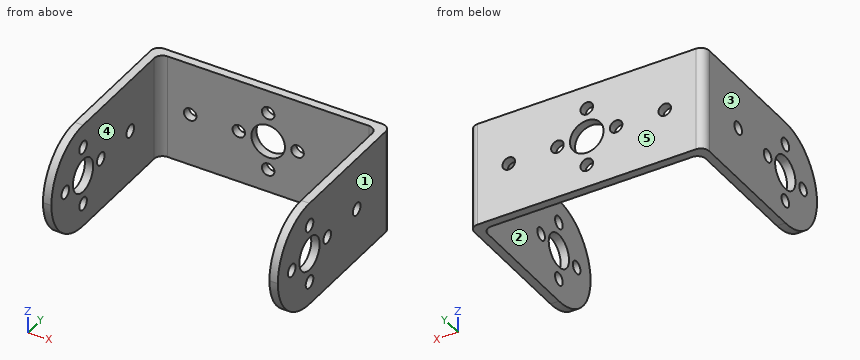
from build123d import *

# Parameters (mm, degrees)
SKETCH_1_W          = 52
SKETCH_1_H          = 25
SKETCH_1_R          = 4
SKETCH_1_R_2        = 1.5
EXTRUDE_1_DEPTH     = 2
SKETCH_2_W          = 2
SKETCH_2_H          = 25
EXTRUDE_2_DEPTH     = 44.5
FILLET_1_R          = 12.5
FILLET_2_R          = 12.5
SKETCH_3_R          = 4
SKETCH_3_R_2        = 1.5
CUT_EXTRUDE_1_DEPTH = 64.5
FILLET_5_R          = 2


with BuildPart() as part:
    # 草图1 → 凸台-拉伸1 (new body)
    with BuildSketch(Plane(origin=(0, 0, 0), x_dir=(1, 0, 0), z_dir=(0, 1, 0))):
        with Locations((-26, 12.5)):
            Rectangle(SKETCH_1_W, SKETCH_1_H)
        with Locations(Location((-26, 12.5, 0), (0, 0, 270))):
            Circle(SKETCH_1_R, mode=Mode.SUBTRACT)
        with Locations(Location((-26, 5.5, 0), (0, 0, 270))):
            Circle(SKETCH_1_R_2, mode=Mode.SUBTRACT)
        with Locations(Location((-33, 12.5, 0), (0, 0, 270))):
            Circle(SKETCH_1_R_2, mode=Mode.SUBTRACT)
        with Locations(Location((-26, 19.5, 0), (0, 0, 270))):
            Circle(SKETCH_1_R_2, mode=Mode.SUBTRACT)
        with Locations(Location((-19, 12.5, 0), (0, 0, 270))):
            Circle(SKETCH_1_R_2, mode=Mode.SUBTRACT)
        with Locations(Location((-7.4, 12.5, 0), (0, 0, 270))):
            Circle(SKETCH_1_R_2, mode=Mode.SUBTRACT)
        with Locations(Location((-44.6, 12.5, 0), (0, 0, 270))):
            Circle(SKETCH_1_R_2, mode=Mode.SUBTRACT)
    extrude(amount=EXTRUDE_1_DEPTH)

    # 草图2 → 凸台-拉伸2 (add)
    with BuildSketch(Plane(origin=(0, 2, 0), x_dir=(1, 0, 0), z_dir=(0, 1, 0))):
        with Locations((-53, 12.5)):
            Rectangle(SKETCH_2_W, SKETCH_2_H)
        with Locations((1, 12.5)):
            Rectangle(SKETCH_2_W, SKETCH_2_H)
    extrude(amount=-EXTRUDE_2_DEPTH)

    # 圆角1
    fillet_1_edges = [part.edges().sort_by_distance(p)[0] for p in [
        (-53, -42.5, -25),
        (-53, -42.5, 0),
    ]]
    fillet(fillet_1_edges, radius=FILLET_1_R - 0.0001)  # a hair under: the kernel refuses the full size

    # 圆角2
    fillet_2_edges = [part.edges().sort_by_distance(p)[0] for p in [
        (1, -42.5, -25),
        (1, -42.5, 0),
    ]]
    fillet(fillet_2_edges, radius=FILLET_2_R - 0.0001)  # a hair under: the kernel refuses the full size

    # 草图3 → 切除-拉伸1 (cut)
    with BuildSketch(Plane(origin=(2, 0, 0), x_dir=(0, 0, -1), z_dir=(1, 0, 0))):
        with Locations((12.5, -30)):
            Circle(SKETCH_3_R)
        with Locations((12.5, -23)):
            Circle(SKETCH_3_R_2)
        with Locations((19.5, -30)):
            Circle(SKETCH_3_R_2)
        with Locations((12.5, -37)):
            Circle(SKETCH_3_R_2)
        with Locations((5.5, -30)):
            Circle(SKETCH_3_R_2)
        with Locations((12.5, -11.4)):
            Circle(SKETCH_3_R_2)
    extrude(amount=-CUT_EXTRUDE_1_DEPTH, mode=Mode.SUBTRACT)

    # 圆角5
    fillet_5_edges = [part.edges().sort_by_distance(p)[0] for p in [
        (-54, 2, -12.5),
        (-52, 0, -12.5),
        (2, 2, -12.5),
        (0, 0, -12.5),
    ]]
    fillet(fillet_5_edges, radius=FILLET_5_R)


solid = part.part
Design review of the part built by this model. Coordinates are the model's own, in mm. Face numbers are marked on the shaded views. A direction names the side the tool comes from. Round coordinates to 2 decimals unless told otherwise and drop trailing zeros. Write each loop counter-clockwise with the first axis right and the second up, starting at its lowest first coordinate (ties: lowest second). Pieces come first, ordered by that corner, then holes. Notation, with made-up numbers: (-14.5, 38) -> (0.5, 38) arc R29 ccw to (0.5, 77) -> close; hole circle Ø9 at (87, 26). An arc over 180 degrees is marked (long way). One line per item, written item: value. Start each with the question number.
Q1. Add section C-C (x = -44.6). Give the boundary of the cut face in (y, z), then the cut area to 3 significant figures.
Q2. Tool access review of the marked faces 4 and 5: name each direction out of +Z, -Z, +X, -X, +Y, -Y from which nothing blocks a thin tool from reaching the whole face with its end or side.
Q3. Add section D-D (z = -5.5). Give the boundary of the cut face in (x, y).
Q4. Add section B-B (y = -14). Give the boundary of the cut face in (x, z).
Q5. Insertion check: P1, Ø4, axis at x = -48, z = -10.5, coming from the -Y side. The pin has a flat end and moves straight along its axis. Give the tip position at first contact, or say it passes through.
Q6. The part is to be moulded in two halves that separate along X. For the marked faces 1, 2 and 3, say which applies: pulls with the +X half, pulls with the -X half, needs draft (parallel to the pull), parting line crosses it, or undercut.
Q7. Add section A-A (y = -23). Give the boundary of the cut face in (x, z).
Q8. To check wall thickness, follow probe 1 along X at (y, z) = (-25.5, -2.5); probe 2 along Y at (x, z) = (-7.5, -14.5); probe 3 along Y at (x, z) = (1.3, -19.5). State the ranges of each line that lie inside material, in increasing order.
Response:
1. outline: (0, -25) -> (2, -25) -> (2, -14) -> (0, -14) -> close; (0, -11) -> (2, -11) -> (2, 0) -> (0, 0) -> close
1. area: 44.0 mm^2
2. face 4: +Z, -Z, -Y
2. face 5: +Z, -Z, +X, -X, +Y
3. outline: (-54, -40.36) -> (-52, -40.36) -> (-52, -31.5) -> (-54, -31.5) -> close; (-54, -28.5) -> (-52, -28.5) -> (-52, -2) arc R2 cw to (-50, 0) -> (-27.5, 0) -> (-27.5, 2) -> (-52, 2) arc R2 ccw to (-54, 0) -> close; (-24.5, 0) -> (-2, 0) arc R2 cw to (0, -2) -> (0, -28.5) -> (2, -28.5) -> (2, 0) arc R2 ccw to (0, 2) -> (-24.5, 2) -> close; (0, -40.36) -> (2, -40.36) -> (2, -31.5) -> (0, -31.5) -> close
4. outline: (-54, -25) -> (-52, -25) -> (-52, 0) -> (-54, 0) -> close; (0, -25) -> (2, -25) -> (2, 0) -> (0, 0) -> close
5. P1: stops at y = 0
6. face 1: pulls with the +X half
6. face 2: undercut
6. face 3: pulls with the -X half
7. outline: (-54, -25) -> (-52, -25) -> (-52, -14) -> (-54, -14) -> close; (-54, -11) -> (-52, -11) -> (-52, 0) -> (-54, 0) -> close; (0, -25) -> (2, -25) -> (2, -14) -> (0, -14) -> close; (0, -11) -> (2, -11) -> (2, 0) -> (0, 0) -> close
8. probe 1: x = -54 to -52, 0 to 2
8. probe 2: y = 0 to 2
8. probe 3: y = -40.36 to -31.5, -28.5 to 1.52
